from build123d import *

# Parameters (mm, degrees)
F1_DEPTH = 6.35
F2_R     = 6.3499
F0_R     = 5.08
F3_DEPTH = 6.35
F0_R_2   = 4.826
F4_DEPTH = 6.35
F5_DEPTH = 6.35


# Not quite as in the source:
# - a fillet or chamfer is up to 0.001 mm smaller than in the source, because OpenCascade refuses the exact size


with BuildPart() as f1:
    # F0 (on Front) → F1 (new body, symmetric)
    with BuildSketch(Plane.XZ):
        with BuildLine():
            Line((25.4, 6.35), (-25.4, 6.35))
            ThreePointArc((-25.4, 6.35), (-23.7445407024, 3.3649028089), (-23.171147458, 0))
            ThreePointArc((-23.171147458, 0), (-23.7445407024, -3.3649028089), (-25.4, -6.35))
            Line((-25.4, -6.35), (25.4, -6.35))
            ThreePointArc((25.4, -6.35), (23.171147458, 0), (25.4, 6.35))
        make_face()
    extrude(amount=F1_DEPTH, both=True)

    # F2 (radius 6.35 in the source; OpenCascade refuses exactly that, so slightly less here)
    f2_edges = [f1.edges().sort_by_distance(p)[0] for p in [
        (0, -6.35, 6.35),
        (0, 6.35, 6.35),
        (0, -6.35, -6.35),
        (0, 6.35, -6.35),
    ]]
    fillet(f2_edges, radius=F2_R)

    # F0 (on Front) → F3 (join)
    with BuildSketch(Plane.XZ):
        with BuildLine():
            ThreePointArc((43.491147458, 0), (36.6960502669, 9.5866067556), (25.4, 6.35))
            Line((25.4, 6.35), (25.4, -6.35))
            ThreePointArc((25.4, -6.35), (36.6960502669, -9.5866067556), (43.491147458, 0))
        make_face()
        with Locations((33.331147458, 0)):
            Circle(F0_R, mode=Mode.SUBTRACT)
        with BuildLine():
            Line((25.4, -6.35), (25.4, 6.35))
            ThreePointArc((25.4, 6.35), (23.171147458, 0), (25.4, -6.35))
        make_face()
    extrude(amount=F3_DEPTH)

    # F0 (on Front) → F4 (join)
    with BuildSketch(Plane.XZ):
        with BuildLine():
            Line((-25.4, -6.35), (-25.4, 6.35))
            ThreePointArc((-25.4, 6.35), (-43.491147458, 0), (-25.4, -6.35))
        make_face()
        with Locations((-33.331147458, 0)):
            Circle(F0_R_2, mode=Mode.SUBTRACT)
        with BuildLine():
            ThreePointArc((-23.171147458, 0), (-23.7445407024, 3.3649028089), (-25.4, 6.35))
            Line((-25.4, 6.35), (-25.4, -6.35))
            ThreePointArc((-25.4, -6.35), (-23.7445407024, -3.3649028089), (-23.171147458, 0))
        make_face()
    extrude(amount=-F4_DEPTH)

    # F0 (on Front) → F5 (join, symmetric)
    with BuildSketch(Plane.XZ):
        with Locations((-33.331147458, 0)):
            Circle(F0_R_2)
    extrude(amount=F5_DEPTH, both=True)


solid = f1.part
Check sheet for the modelled part. Datum: model origin and axes. Units: mm. A direction names the side the tool comes from. Give positions to 0.01 mm unless a question says otherwise; leave off trailing zeros. Loops run counter-clockwise (first coordinate to the right, second up) from the corner with the lowest first, then second, coordinate; pieces in that order, holes last. Notation, with made-up numbers: M -21,77.5 L 10,77.5 A19 cw 10,88.5 Z; hole C -22.5,26 d6. An arc over 180 degrees is marked long. Use a Markdown table: item, result. Add a question column.
Q1. Sectioned sample at D-D, the plane x = 32. Record the cut outline in (y, z), then the cut area to 3 significant figures.
Q2. Sectioned sample at B-B, the plane z = -8.25. Record the cut outline in (x, y).
Q3. Mould release check, pull along Z, two halves, no side actions. Record for faces 6 (the cylindrical face through (-0.36, -4.44, 4.54)), 7 (the cylindrical face through (-23.17, -2.51, 0.1)), 8 (the cylindrical face through (0.36, -4.44, -4.54)), 9 (the cylindrical face through (-28.873, -3.219, -1.848)): pulls with the +Z half, pulls with the -Z half, needs draft (parallel to the pull), parting line crosses it, or undercut.
Q4. Sectioned sample at A-A, the plane y = -4.75. Record the cut outline in (x, z).
Q5. Scan lines: line 1 along Y through (x, z) = (-39, -5.5); line 2 along X through (y, z) = (-1.25, -1.25); line 3 along X through (y, z) = (-5.5, 3.25). Record each from-to range of solid material in increasing order. Write a range as [from, to].
Q6. Go/stop test with flat-tipped pins: pin 1 (3 mm diameter, centred on x = 11.5, y = 2.5, fed in from -Z); pin 2 (1 mm diameter, centred on y = -4.5, z = 2, fed in from +X); pin 3 (4 mm diameter, centred on x = -30.5, y = -5, fed in from -Z). Record where each tip stops, or that it passes through.
Q7. Tool access check on faces 1 (the flat face through (-28.96, 0, 2.4)), 2 (the flat face through (-33, 6.35, 0)), 3 (the cylindrical face through (23.17, 2.42, -0.1)), 4 (the cylindrical face through (0.36, 4.44, -4.54)), 5 (the cylindrical face through (-0.36, 4.44, 4.54)). Record the directions out of +Z, -Z, +X, -X, +Y, -Y that give a thin tool (end or side, any length) a straight path to the whole face; none if there is none.
Verdict:
| question | item | result |
|---|---|---|
| 1 | outline | M -6.35,-10.07 L 0,-10.07 L 0,-4.9 L -6.35,-4.9 Z; M -6.35,4.9 L 0,4.9 L 0,10.07 L -6.35,10.07 Z |
| 1 | area | 65.7 mm^2 |
| 2 | outline | M -39.26,0 L -27.4,0 L -27.4,6.35 L -39.26,6.35 Z; M 27.4,-6.35 L 39.26,-6.35 L 39.26,0 L 27.4,0 Z |
| 3 | face 6 | pulls with the +Z half |
| 3 | face 7 | undercut |
| 3 | face 8 | pulls with the -Z half |
| 3 | face 9 | parting line crosses it |
| 4 | outline | C -33.33,0 d9.65; M -24.09,-4.21 L 24.09,-4.21 A10.16 ccw long 24.09,4.21 L -24.09,4.21 A10.16 cw Z; hole C 33.33,0 d10.16 |
| 5 | line 1 | [0, 6.35] |
| 5 | line 2 | [-37.99, -28.67], [-23.25, 28.41], [38.25, 43.41] |
| 5 | line 3 | [-36.9, -29.76], [23.7, 29.43], [37.24, 42.96] |
| 6 | pin 1 | z = -6.27 |
| 6 | pin 2 | x = 43.38 |
| 6 | pin 3 | z = -4.75 |
| 7 | face 1 | -Y |
| 7 | face 2 | +Z, -Z, +X, -X, +Y |
| 7 | face 3 | +X, +Y |
| 7 | face 4 | -Z, +X, +Y |
| 7 | face 5 | +Z, +X, +Y |
